Input: part model. Units: mm. Frame: model coordinates. A direction names the side the tool comes from. Coordinates: 2 decimals unless noted, no trailing zeros. Order: outer loops, then holes, each group sorted by start corner. A loop starts at its lowest first (then second) coordinate and runs counter-clockwise, first axis right, second up. Notation, with made-up numbers: (86.25, 23) - (97.25, 23) arc R24 ccw to (97.25, 40) - close; hole circle Ø2 at (-4.75, 31). An arc over 180 degrees is marked (long way). One line per question, with ' | ' between items. Start each with the question number.
```python
from build123d import *

# Parameters (mm, degrees)
SKETCH1_R                = 2.5
BOSS_EXTRUDE1_DEPTH      = 1.5
BOSS_EXTRUDE2_DEPTH      = 4
BOSS_EXTRUDE2_DEPTH_BACK = 2
SKETCH2_R                = 6
SKETCH3_R                = 9
SKETCH3_R_2              = 6
BOSS_EXTRUDE3_DEPTH      = 5
FILLET1_R                = 5


with BuildPart() as part:
    # Sketch1 → Boss-Extrude1 (new body)
    with BuildSketch(Plane(origin=(0, 0, 0), x_dir=(1, 0, 0), z_dir=(0, 1, 0))):
        with BuildLine():
            Line((-13, -18), (13, -18))
            ThreePointArc((13, -18), (16.535533906, -16.535533906), (18, -13))
            Line((18, -13), (18, 13))
            ThreePointArc((18, 13), (16.535533906, 16.535533906), (13, 18))
            Line((13, 18), (-13, 18))
            ThreePointArc((-13, 18), (-16.535533906, 16.535533906), (-18, 13))
            Line((-18, 13), (-18, -13))
            ThreePointArc((-18, -13), (-16.535533906, -16.535533906), (-13, -18))
        make_face()
        with Locations(Location((13.435028843, 13.435028843, 0), (0, 0, 270))):
            Circle(SKETCH1_R, mode=Mode.SUBTRACT)
        with Locations(Location((-13.435028843, -13.435028843, 0), (0, 0, 270))):
            Circle(SKETCH1_R, mode=Mode.SUBTRACT)
        with Locations(Location((-13.435028843, 13.435028843, 0), (0, 0, 270))):
            Circle(SKETCH1_R, mode=Mode.SUBTRACT)
        with Locations(Location((13.435028843, -13.435028843, 0), (0, 0, 270))):
            Circle(SKETCH1_R, mode=Mode.SUBTRACT)
    extrude(amount=BOSS_EXTRUDE1_DEPTH)

    # Sketch2 → Boss-Extrude2 (add, two sides: drawn at the far end of the back side and taken through both)
    with BuildSketch(Plane.XZ.offset(-BOSS_EXTRUDE2_DEPTH_BACK)):
        with Locations(Location((0, 0, 0), (0, 0, 270))):
            Circle(SKETCH2_R)
    extrude(amount=BOSS_EXTRUDE2_DEPTH + BOSS_EXTRUDE2_DEPTH_BACK)

    # Sketch3 → Boss-Extrude3 (add)
    with BuildSketch(Plane(origin=(0, -3, 0), x_dir=(-1, 0, 0), z_dir=(0, -1, 0))):
        with Locations(Location((0, 0, 0), (0, 0, 90))):
            Circle(SKETCH3_R)
        with Locations(Location((0, 0, 0), (0, 0, 90))):
            Circle(SKETCH3_R_2, mode=Mode.SUBTRACT)
    extrude(amount=BOSS_EXTRUDE3_DEPTH)

    # Fillet1
    # the kernel refuses this fillet: 5 mm, written as the material it takes off along each edge
    with BuildSketch(Plane(origin=(0, -3, 0), x_dir=(0, 0, -1), z_dir=(-1, 0, 0))) as fillet1_piece_1:
        with BuildLine():
            CenterArc((4, 4.582575695), FILLET1_R, 293.578178478, 66.421821522)
            Line((9, 4.582575695), (9.1, 4.582575695))
            Line((9.1, 4.582575695), (9.1, 0))
            Line((9.1, 0), (9, -0.1))
            ThreePointArc((9, -0.1), (7.5, -0.1), (6.04, -0.091651514))
            Line((6.04, -0.091651514), (6, 0))
        make_face()
    revolve(axis=Axis((0, -3, 0), (0, -1, 0)), mode=Mode.SUBTRACT)


solid = part.part
```
(1) Reachability of faces 1 (the face through (-8, 1.5, 0)), 2 (the face through (0, -4, 0)), 3 (the face through (-8, 0, 0)), 4 (the face through (-16, 1, -17)) from +Z, -Z, +X, -X, +Y, -Y: full face, straight path, thin tool, end or side. Return the list, or none.
(2) Material intervals for line 1 along X through (y, z) = (0.5, -12); line 2 along X through (y, z) = (-5.25, -0.5); line 3 along Y through (x, z) = (2, -1), sorted ascending. Write a range as from..to.
(3) Pin query (flat end, axial travel): pin 1 (6 mm diameter, centred on x = 6.5, z = 13.5, fed in from +Y); pin 2 (4.5 mm diameter, centred on x = 13.44, z = -13.44, fed in from -Y); pin 3 (8 mm diameter, centred on x = -13.44, z = -13.44, fed in from -Y). Return the tip coordinate at first contact, or that it passes through.
(4) Draft query along Y for faces 5 (the face through (-6, -8, -2)), 6 (the face through (1.802, -1.479, -5.723)), 7 (the face through (0, 2, 0)), 8 (the face through (16, 1, 17)). Return one class per face: +Y half, -Y half, draft (parallel to the pull), parting line (faces both ways), or undercut.
(5) Section B-B (z = -13.5). Output: boundary loops of the cut face in (x, y).
(6) Section D-D (y = -1.75). Output: boundary loops of the cut face in (x, z), then the cut area to 3 significant figures.
(7) Section C-C (x = 15). Output: boundary loops of the cut face in (y, z), then the cut area to 3 significant figures.
(8) Section A-A (y = 1). Output: boundary loops of the cut face in (x, z).
Worked answers:
1) face 1: +Y | face 2: -Y | face 3: none | face 4: -Z, -X, +Y, -Y
2) line 1: x = -18..-15.48, -11.39..11.39, 15.48..18 | line 2: x = -8.41..-5.98, 5.98..8.41 | line 3: y = -4..2
3) pin 1: stops at y = 1.5 | pin 2: passes through | pin 3: stops at y = 0
4) face 5: -Y half | face 6: undercut | face 7: +Y half | face 8: draft
5) outline: (-17.97, 0) - (-15.93, 0) - (-15.93, 1.5) - (-17.97, 1.5) - close; (-10.94, 0) - (10.94, 0) - (10.94, 1.5) - (-10.94, 1.5) - close; (15.93, 0) - (17.97, 0) - (17.97, 1.5) - (15.93, 1.5) - close
6) outline: circle Ø12 at (0, 0) | area: 113 mm²
7) outline: (0, -17.58) - (1.5, -17.58) - (1.5, -15.38) - (0, -15.38) - close; (0, -11.49) - (1.5, -11.49) - (1.5, 11.49) - (0, 11.49) - close; (0, 15.38) - (1.5, 15.38) - (1.5, 17.58) - (0, 17.58) - close | area: 41.1 mm²
8) outline: (-18, -13) arc R5 ccw to (-13, -18) - (13, -18) arc R5 ccw to (18, -13) - (18, 13) arc R5 ccw to (13, 18) - (-13, 18) arc R5 ccw to (-18, 13) - close; hole circle Ø5 at (-13.44, -13.44); hole circle Ø5 at (-13.44, 13.44); hole circle Ø5 at (13.44, -13.44); hole circle Ø5 at (13.44, 13.44)
